The model under review builds one solid part; all positions refer to its coordinate system, in mm. A direction names the side the tool comes from. Give positions to 0.01 mm unless a question says otherwise; leave off trailing zeros. Loops run counter-clockwise (first coordinate to the right, second up) from the corner with the lowest first, then second, coordinate; pieces in that order, holes last. Notation, with made-up numbers: (-17, 70.25) - (31, 70.25) arc R21 cw to (31, 89.25) - close; hole circle Ø6 at (4, 30.5). An arc over 180 degrees is marked (long way). Answer as a JSON object with one key per item and string values.
from build123d import *

# Parameters (mm, degrees)
F0_W     = 101.6
F0_H     = 101.6
F1_DEPTH = 101.6
F2_W     = 76.2
F2_H     = 76.2
F3_DEPTH = 168.91
F4_W     = 25.4
F4_H     = 54.637392
F5_DEPTH = 81.026
F7_DEPTH = 51.562


with BuildPart() as f1:
    # F0 (on Top) → F1 (new body)
    with BuildSketch(Plane.XY):
        with Locations((-50.8, -50.8)):
            Rectangle(F0_W, F0_H)
    extrude(amount=F1_DEPTH)

    # F2 (on face) → F3 (cut)
    with BuildSketch(Plane.XZ.offset(101.6)):
        with Locations((-63.5, 63.5)):
            Rectangle(F2_W, F2_H)
    extrude(amount=-F3_DEPTH, mode=Mode.SUBTRACT)

    # F4 (on face) → F5 (cut)
    with BuildSketch(Plane.XY.offset(25.4)):
        with Locations((-88.9, -48.881304)):
            Rectangle(F4_W, F4_H)
    extrude(amount=-F5_DEPTH, mode=Mode.SUBTRACT)

    # F6 (on face) → F7 (cut)
    with BuildSketch(Plane(origin=(-25.4, 0, 0), x_dir=(0, -1, 0), z_dir=(-1, 0, 0))):
        Polygon((25.4, 101.6), (0, 101.6), (0, 76.2), align=None)
        Polygon((101.6, 101.6), (76.2, 101.6), (101.6, 76.2), align=None)
        Polygon((76.2, 101.6), (25.4, 101.6), (25.4, 76.2), (25.4, 50.8), (76.2, 50.8), (76.2, 76.2), align=None)
    extrude(amount=-F7_DEPTH, mode=Mode.SUBTRACT)


solid = f1.part
Q1. Consider section D-D, the plane y = -49. State the section outline as (x, z) points, plus the area to 3 significant figures.
Results:
{"outline": "(-76.2, 0) - (0, 0) - (0, 50.8) - (-25.4, 50.8) - (-25.4, 25.4) - (-76.2, 25.4) - close", "area": "2,580 mm^2"}
Q2. To check wall thickness, follow probe 1 along Z at (x, y) = (-48.5, -15.5); probe 2 along X at (y, z) = (-43, 36); probe 3 along X at (y, z) = (-39, 19). State the ranges of each line that lie inside material, in increasing order. Write a range as [from, to].
Results:
{"probe 1": "z = [0, 25.4]", "probe 2": "x = [-25.4, 0]", "probe 3": "x = [-76.2, 0]"}
Q3. Consider section B-B, the plane x = -82. State the section outline as (y, z) points, plus the area to 3 significant figures.
Results:
{"outline": "(-101.6, 0) - (-76.2, 0) - (-76.2, 25.4) - (-101.6, 25.4) - close; (-21.56, 0) - (0, 0) - (0, 25.4) - (-21.56, 25.4) - close", "area": "1,190 mm^2"}
Q4. The part is to be moulded in two halves that separate along Y. For faces 5 (the face through (-13, -76.2, 76)), 6 (the face through (-52, -50, 0)), 7 (the face through (-12.9, -88.7, 89.1)), say which applies: +Y half, -Y half, draft (parallel to the pull), parting line (faces both ways), or undercut.
Results:
{"face 5": "undercut", "face 6": "draft", "face 7": "-Y half"}
Q5. Clearance check with flat-ended pins moving along their axes: pin 1 Ø23 at (x, y) = (-66.5, -26.5) entering from +Z; pin 2 Ø7.5 at (y, z) = (-40.5, 14) entering from -X; pin 3 Ø12.5 at (x, y) = (-11, -57) entering from +Z. State where each tip first meets the part, or that it passes through.
Results:
{"pin 1": "stops at z = 25.4", "pin 2": "stops at x = -76.2", "pin 3": "stops at z = 50.8"}
Q6. Consider section C-C, the plane x = -13. State the section outline as (y, z) points.
Results:
{"outline": "(-101.6, 0) - (0, 0) - (0, 76.2) - (-25.4, 101.6) - (-25.4, 50.8) - (-76.2, 50.8) - (-76.2, 101.6) - (-101.6, 76.2) - close"}
Q7. Consider section A-A, the plane z = 53.5. State the section outline as (x, y) points.
Results:
{"outline": "(-25.4, -101.6) - (0, -101.6) - (0, -76.2) - (-25.4, -76.2) - close; (-25.4, -25.4) - (0, -25.4) - (0, 0) - (-25.4, 0) - close"}
Q8. For faces 1 (the face through (-76.2, -49, 13)), 2 (the face through (-13, -25.4, 77)), 3 (the face through (-25.4, -52, 46)), 4 (the face through (-12.9, -12.5, 88.7)), list the 3-axis set-ups (+Z, -Z, +X, -X, +Y, -Y) from which the entire face can be reached by the end or side of a thin tool; tool diameter is ignored.
Results:
{"face 1": "+Z, -Z, -X", "face 2": "+Z, +X, -X", "face 3": "+Z, -X, +Y, -Y", "face 4": "+Z, +X, -X, +Y"}
